```python
from build123d import *

# Parameters (mm, degrees)
F0_W      = 25.4
F0_H      = 2.54
F0_H_2    = 1.524
F1_DEPTH  = 13.8684
F2_DEPTH  = 2.54
F3_DEPTH  = 1.397
F4_DEPTH  = 0.127
F5_DEPTH  = 3.6576
F6_W      = 13.97
F6_H      = 13.8684
F7_DEPTH  = 1.5875
F8_W      = 13.97
F8_H      = 1.5875
F9_DEPTH  = 1.5875
F10_W     = 13.97
F10_H     = 1.5875
F11_DEPTH = 1.5875
F12_DEPTH = 12.7


with BuildPart() as f1:
    # F0 (on Front) → F1 (new body)
    with BuildSketch(Plane.XZ):
        Polygon((12.7, 12.7), (-12.7, 12.7), (-12.7, -4.10832325), (-12.7, -8.636), (12.7, -8.636), align=None)
        with BuildLine():
            ThreePointArc((-4.0682750421, 8.452909583), (-3.8265239697, 8.4581987178), (-3.584766021, 8.4532338248))
            Line((-3.584766021, 8.4532338248), (3.8188760303, 8.4581987178))
            ThreePointArc((3.8188760303, 8.4581987178), (9.5249996895, 2.7577817272), (3.8226394845, -2.9463999997))
            Line((3.8226394845, -2.9463999997), (-3.7923413869, -2.9463191859))
            ThreePointArc((-3.7923413869, -2.9463191859), (-3.8227605155, -2.9463999997), (-3.8531796423, -2.9463185403))
            ThreePointArc((-3.8531796423, -2.9463185403), (-9.5239851182, 2.6483207685), (-4.0682750421, 8.452909583))
        make_face(mode=Mode.SUBTRACT)
        with Locations((0, -9.906)):
            Rectangle(F0_W, F0_H)
        with Locations((0, -11.938)):
            Rectangle(F0_W, F0_H_2)
    extrude(amount=F1_DEPTH)

    # F0 (on Front) → F2 (cut)
    with BuildSketch(Plane.XZ):
        with Locations((0, -9.906)):
            Rectangle(F0_W, F0_H)
    extrude(amount=F2_DEPTH, mode=Mode.SUBTRACT)

    # F3 (add): a face of the model
    f3_faces = [f1.faces().sort_by_distance(p)[0] for p in [
        (12.7, -7.0398753731, 0.1848134328),
    ]]
    extrude(f3_faces, amount=F3_DEPTH)

    # F4 (cut): a face of the model
    f4_faces = [f1.faces().sort_by_distance(p)[0] for p in [
        (-12.7, -7.0398753731, 0.1848134328),
    ]]
    extrude(f4_faces, amount=-F4_DEPTH, mode=Mode.SUBTRACT)

    # F5 (add): a face of the model
    f5_faces = [f1.faces().sort_by_distance(p)[0] for p in [
        (0.762, -6.9342, -12.7),
    ]]
    extrude(f5_faces, amount=F5_DEPTH)

    # F6 (on face) → F7 (join)
    with BuildSketch(Plane.XY.offset(12.7)):
        with Locations((7.112, -6.9342)):
            Rectangle(F6_W, F6_H)
    extrude(amount=F7_DEPTH)

    # F8 (on face) → F9 (join)
    with BuildSketch(Plane.XZ.offset(13.8684)):
        with Locations((7.112, 13.49375)):
            Rectangle(F8_W, F8_H)
    extrude(amount=F9_DEPTH)

    # F10 (on face) → F11 (join)
    with BuildSketch(Plane(origin=(0, 0, 0), x_dir=(-1, 0, 0), z_dir=(0, 1, 0))):
        with Locations((-7.112, 13.49375)):
            Rectangle(F10_W, F10_H)
    extrude(amount=F11_DEPTH)

    # F12 (add, through all): a face of the model
    f12_faces = [f1.faces().sort_by_distance(p)[0] for p in [
        (0.127, -6.9342, 13.49375),
    ]]
    extrude(f12_faces, amount=F12_DEPTH)


solid = f1.part
```
Read the model definition and answer for the solid it produces. Units are mm, in the model's axes. A direction names the side the tool comes from. Give positions to 0.01 mm unless a question says otherwise; leave off trailing zeros. Order: outer loops, then holes, each group sorted by start corner. A loop starts at its lowest first (then second) coordinate and runs counter-clockwise, first axis right, second up.
(1) Find section C-C (z = 3). Give the vertices of the cut face in (x, y), plus the area to 3 significant figures.
(2) Find section B-B (x = -0.5). Give the vertices of the cut face in (y, z), plus the area to 3 significant figures.
(3) Find section D-D (x = -10). Give the vertices of the cut face in (y, z), plus the area to 3 significant figures.
(4) Find section A-A (y = -3.5). Give the vertices of the cut face in (x, z).
(5) For faces 5 (the flat face through (1, 0, -5)), 6 (the flat face through (1, -13.868, -5)), 7 (the flat face through (1, -1, -8.636)), determine the directions among +Z, -Z, +X, -X, +Y, -Y from which every point of the face is accessible in a straight line to the end or side of a thin tool.
(6) For a pull along X with two mould halves and no side action, classify faces 1 (the cylindrical face through (9.524, -6.837, 2.883)), 2 (the flat face through (14.097, -7, -1)), 3 (the flat face through (-12.573, -7, -1)), 4 (the flat face through (1, -7, -16.358)) as released by +X, released by -X, zero draft, split by the parting line, or undercut.
(7) Given pin 1 (1.3 mm diameter, centred on x = -4, y = 1, fed in from -Z); pin 2 (5 mm diameter, centred on x = -7, z = -1.5, fed in from +Y); pin 3 (3 mm diameter, centred on x = 9, z = -9.5, fed in from -Y), each flat-ended and moving along its own axis, determine where each tip first touches the part or whether it passes through.
(8) Straight lines are drawn through the part: L1, parallel to Z at x = -3, y = -8.25; L2, parallel to Z at x = -9.75, y = -0.5; L3, parallel to X at y = -4.25, z = 3. For each, find the intervals that lie inside material, in ascending order.
Result sheet:
1. outline: (-12.57, -13.87) - (-9.52, -13.87) - (-9.52, 0) - (-12.57, 0) - close; (9.52, -13.87) - (14.1, -13.87) - (14.1, 0) - (9.52, 0) - close
1. area: 106 mm2
2. outline: (-15.46, 12.7) - (-13.87, 12.7) - (-13.87, 8.46) - (0, 8.46) - (0, 12.7) - (1.59, 12.7) - (1.59, 14.29) - (-15.46, 14.29) - close; (-13.87, -16.36) - (0, -16.36) - (0, -11.18) - (-2.54, -11.18) - (-2.54, -8.64) - (0, -8.64) - (0, -2.95) - (-13.87, -2.95) - close
2. area: 265 mm2
3. outline: (-15.46, 12.7) - (-13.87, 12.7) - (-13.87, -16.36) - (0, -16.36) - (0, -11.18) - (-2.54, -11.18) - (-2.54, -8.64) - (0, -8.64) - (0, 12.7) - (1.59, 12.7) - (1.59, 14.29) - (-15.46, 14.29) - close
3. area: 424 mm2
4. outline: (-12.57, -16.36) - (14.1, -16.36) - (14.1, 14.29) - (-12.57, 14.29) - close; hole (-3.85, -2.95) arc R5.7 ccw to (-3.79, -2.95) - (3.82, -2.95) arc R5.7 ccw to (3.82, 8.46) - (-3.58, 8.45) arc R5.7 ccw (long way) to start
5. face 5: -Z, +X, -X, +Y
5. face 6: -Z, +X, -X, -Y
5. face 7: +X, -X, +Y
6. face 1: undercut
6. face 2: released by +X
6. face 3: released by -X
6. face 4: zero draft
7. pin 1: stops at z = 12.7
7. pin 2: stops at y = 0
7. pin 3: stops at y = -13.87
8. L1: z = -16.36 to -2.95, 8.45 to 14.29
8. L2: z = -16.36 to -11.18, -8.64 to 14.29
8. L3: x = -12.57 to -9.52, 9.52 to 14.1
